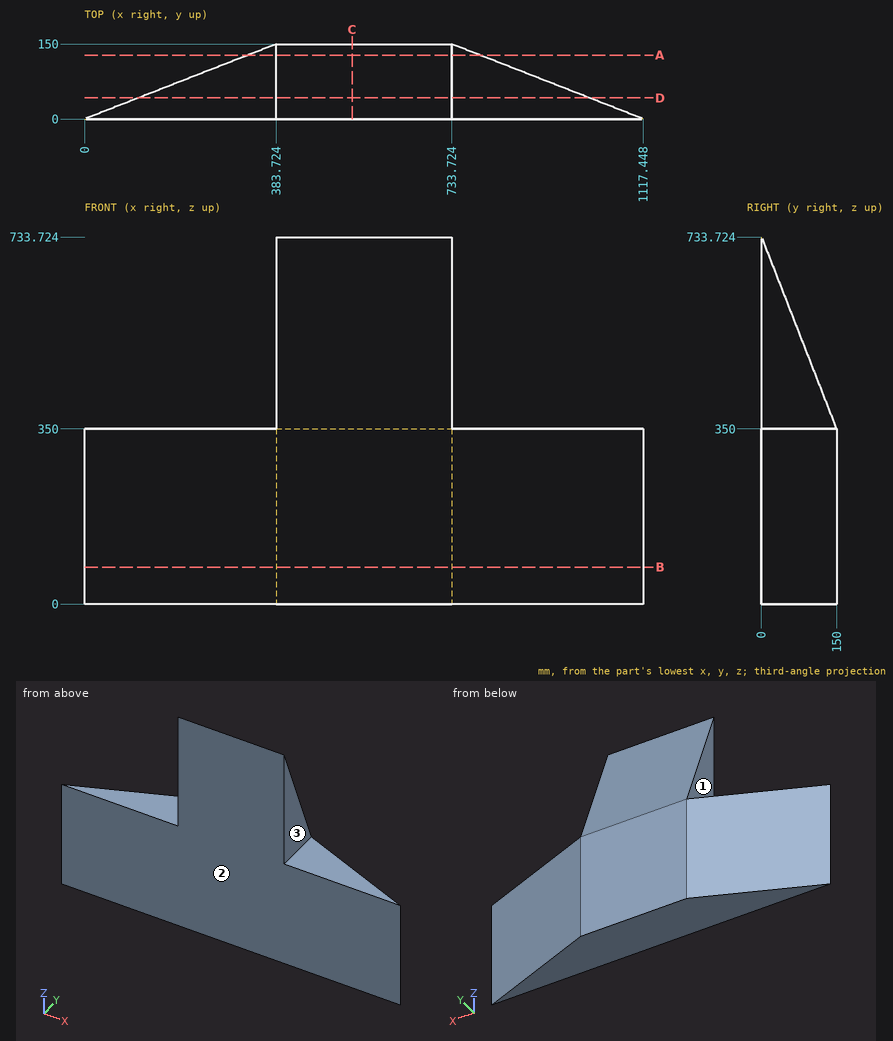
Design review of the part shown in the three views and the two pictorial views. Dimensions are in mm from the part's minimum x, y and z. A direction names the side the tool comes from. Coordinates: 2 decimals unless noted, no trailing zeros. Write each loop counter-clockwise with the first axis right and the second up, starting at its lowest first coordinate (ties: lowest second). Pieces come first, ordered by that corner, then holes.
(1) Add section B-B on z = 74. Give the boundary of the cut face in (x, y), then the cut area to 3 significant figures.
(2) Tool access review of the marked faces 1, 2 and 3: name each direction out of +Z, -Z, +X, -X, +Y, -Y from which nothing blocks a thin tool from reaching the whole face with its end or side.
(3) Add section A-A on y = 128. Give the boundary of the cut face in (x, z), then the cut area to 3 significant figures.
(4) Wall thickness on probe 1 along Z at (x, y) = (382, 11); probe 2 along X at (y, z) = (17, 652); probe 3 along Y at (x, z) = (641.5, 483): over which ranges is each line inside the solid? List them lowest first.
(5) Add section C-C on x = 535. Give the boundary of the cut face in (y, z), then the cut area to 3 significant figures.
(6) Add section D-D on y = 42.5. Give the boundary of the cut face in (x, z).
Answer sheet:
1. outline: (0, 0) - (1117.45, 0) - (733.72, 150) - (383.72, 150) - close
1. area: 110,000 mm2
2. face 1: +Z, -X, +Y, -Y
2. face 2: +Z, -Z, +X, -X, -Y
2. face 3: +Z, +X, +Y, -Y
3. outline: (327.44, 0) - (790, 0) - (790, 350) - (733.72, 350) - (733.72, 406.28) - (383.72, 406.28) - (383.72, 350) - (327.44, 350) - close
3. area: 182,000 mm2
4. probe 1: z = 0 to 350
4. probe 2: x = 383.72 to 733.72
4. probe 3: y = 0 to 98.01
5. outline: (0, 0) - (150, 0) - (150, 350) - (0, 733.72) - close
5. area: 81,300 mm2
6. outline: (108.72, 0) - (1008.73, 0) - (1008.73, 350) - (733.72, 350) - (733.72, 625) - (383.72, 625) - (383.72, 350) - (108.72, 350) - close
